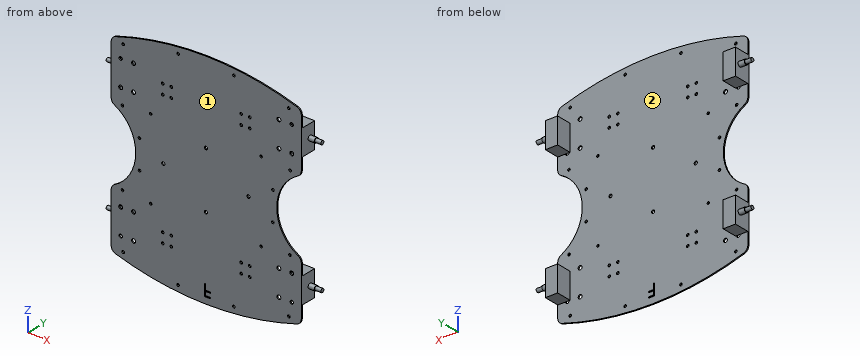
from build123d import *

# Parameters (mm, degrees)
SKETCH1_R           = 2.75
SKETCH1_R_2         = 3.19965974
SKETCH1_R_3         = 2.125
SKETCH1_R_4         = 2.6
SKETCH1_R_5         = 2
BOSS_EXTRUDE1_DEPTH = 2
CUT_EXTRUDE1_DEPTH  = 238.125138886
SKETCH3_R           = 2.125
CUT_EXTRUDE2_DEPTH  = 238.125138886
SKETCH5_W           = 42
SKETCH5_H           = 25
BOSS_EXTRUDE2_DEPTH = 20
BOSS_EXTRUDE3_START = -310
SKETCH5_2_W         = 42
SKETCH5_2_H         = 25
BOSS_EXTRUDE3_DEPTH = 20
SKETCH6_R           = 4
BOSS_EXTRUDE4_DEPTH = 10
SKETCH7_R           = 3
BOSS_EXTRUDE5_DEPTH = 10


with BuildPart() as part:
    # Sketch1 → Boss-Extrude1 (new body)
    with BuildSketch(Plane(origin=(0, 0, 0), x_dir=(1, 0, 0), z_dir=(0, 1, 0))):
        with BuildLine():
            Line((-155, 147.496205723), (-155, 66.522508221))
            ThreePointArc((-155, 66.522508221), (-153.570009292, 61.369359597), (-149.689011853, 57.690001904))
            ThreePointArc((-149.689011853, 57.690001904), (-115, 0), (-149.689011853, -57.690001904))
            ThreePointArc((-149.689011853, -57.690001904), (-153.570009292, -61.369359597), (-155, -66.522508221))
            Line((-155, -66.522508221), (-155, -147.496205723))
            ThreePointArc((-155, -147.496205723), (-153.049591193, -153.429508482), (-147.959183673, -157.048338049))
            ThreePointArc((-147.959183673, -157.048338049), (0, -179.441721715), (147.959183673, -157.048338049))
            ThreePointArc((147.959183673, -157.048338049), (153.049591193, -153.429508482), (155, -147.496205723))
            Line((155, -147.496205723), (155, -66.522508221))
            ThreePointArc((155, -66.522508221), (153.570009292, -61.369359597), (149.689011853, -57.690001904))
            ThreePointArc((149.689011853, -57.690001904), (115, 0), (149.689011853, 57.690001904))
            ThreePointArc((149.689011853, 57.690001904), (153.570009292, 61.369359597), (155, 66.522508221))
            Line((155, 66.522508221), (155, 147.496205723))
            ThreePointArc((155, 147.496205723), (153.049591193, 153.429508482), (147.959183673, 157.048338049))
            ThreePointArc((147.959183673, 157.048338049), (0, 179.441721715), (-147.959183673, 157.048338049))
            ThreePointArc((-147.959183673, 157.048338049), (-153.049591193, 153.429508482), (-155, 147.496205723))
        make_face()
        with Locations(Location((-139.47, 128.51, 0), (0, 0, 270))):
            Circle(SKETCH1_R, mode=Mode.SUBTRACT)
        with Locations(Location((-139.47, 86.51, 0), (0, 0, 270))):
            Circle(SKETCH1_R_2, mode=Mode.SUBTRACT)
        with Locations(Location((139.47, 86.51, 0), (0, 0, 270))):
            Circle(SKETCH1_R_2, mode=Mode.SUBTRACT)
        with Locations(Location((139.47, 128.51, 0), (0, 0, 270))):
            Circle(SKETCH1_R, mode=Mode.SUBTRACT)
        with Locations(Location((139.47, -86.51, 0), (0, 0, 270))):
            Circle(SKETCH1_R_2, mode=Mode.SUBTRACT)
        with Locations(Location((139.47, -128.51, 0), (0, 0, 270))):
            Circle(SKETCH1_R, mode=Mode.SUBTRACT)
        with Locations(Location((-139.47, -86.51, 0), (0, 0, 270))):
            Circle(SKETCH1_R_2, mode=Mode.SUBTRACT)
        with Locations(Location((-139.47, -128.51, 0), (0, 0, 270))):
            Circle(SKETCH1_R, mode=Mode.SUBTRACT)
        with Locations(Location((-70.97, 115.51, 0), (0, 0, 270))):
            Circle(SKETCH1_R_3, mode=Mode.SUBTRACT)
        with Locations(Location((-56.97, 115.51, 0), (0, 0, 270))):
            Circle(SKETCH1_R_3, mode=Mode.SUBTRACT)
        with Locations(Location((-70.97, 99.51, 0), (0, 0, 270))):
            Circle(SKETCH1_R_3, mode=Mode.SUBTRACT)
        with Locations(Location((-56.97, 99.51, 0), (0, 0, 270))):
            Circle(SKETCH1_R_3, mode=Mode.SUBTRACT)
        with Locations(Location((56.97, 99.51, 0), (0, 0, 270))):
            Circle(SKETCH1_R_3, mode=Mode.SUBTRACT)
        with Locations(Location((70.97, 99.51, 0), (0, 0, 270))):
            Circle(SKETCH1_R_3, mode=Mode.SUBTRACT)
        with Locations(Location((56.97, 115.51, 0), (0, 0, 270))):
            Circle(SKETCH1_R_3, mode=Mode.SUBTRACT)
        with Locations(Location((70.97, 115.51, 0), (0, 0, 270))):
            Circle(SKETCH1_R_3, mode=Mode.SUBTRACT)
        with Locations(Location((70.97, -99.51, 0), (0, 0, 270))):
            Circle(SKETCH1_R_3, mode=Mode.SUBTRACT)
        with Locations(Location((56.97, -99.51, 0), (0, 0, 270))):
            Circle(SKETCH1_R_3, mode=Mode.SUBTRACT)
        with Locations(Location((70.97, -115.51, 0), (0, 0, 270))):
            Circle(SKETCH1_R_3, mode=Mode.SUBTRACT)
        with Locations(Location((56.97, -115.51, 0), (0, 0, 270))):
            Circle(SKETCH1_R_3, mode=Mode.SUBTRACT)
        with Locations(Location((-56.97, -99.51, 0), (0, 0, 270))):
            Circle(SKETCH1_R_3, mode=Mode.SUBTRACT)
        with Locations(Location((-70.97, -99.51, 0), (0, 0, 270))):
            Circle(SKETCH1_R_3, mode=Mode.SUBTRACT)
        with Locations(Location((-56.97, -115.51, 0), (0, 0, 270))):
            Circle(SKETCH1_R_3, mode=Mode.SUBTRACT)
        with Locations(Location((-70.97, -115.51, 0), (0, 0, 270))):
            Circle(SKETCH1_R_3, mode=Mode.SUBTRACT)
        with Locations(Location((-118.47, 128.51, 0), (0, 0, 270))):
            Circle(SKETCH1_R_2, mode=Mode.SUBTRACT)
        with Locations(Location((-118.47, 86.51, 0), (0, 0, 270))):
            Circle(SKETCH1_R_2, mode=Mode.SUBTRACT)
        with Locations(Location((118.47, 86.51, 0), (0, 0, 270))):
            Circle(SKETCH1_R_2, mode=Mode.SUBTRACT)
        with Locations(Location((118.47, 128.51, 0), (0, 0, 270))):
            Circle(SKETCH1_R_2, mode=Mode.SUBTRACT)
        with Locations(Location((118.47, -128.51, 0), (0, 0, 270))):
            Circle(SKETCH1_R_2, mode=Mode.SUBTRACT)
        with Locations(Location((118.47, -86.51, 0), (0, 0, 270))):
            Circle(SKETCH1_R_2, mode=Mode.SUBTRACT)
        with Locations(Location((-118.47, -86.51, 0), (0, 0, 270))):
            Circle(SKETCH1_R_2, mode=Mode.SUBTRACT)
        with Locations(Location((-118.47, -128.51, 0), (0, 0, 270))):
            Circle(SKETCH1_R_2, mode=Mode.SUBTRACT)
        with Locations(Location((-0.51, 46.4, 0), (0, 0, 270))):
            Circle(SKETCH1_R_4, mode=Mode.SUBTRACT)
        with Locations(Location((68.99, -0.1, 0), (0, 0, 270))):
            Circle(SKETCH1_R_4, mode=Mode.SUBTRACT)
        with Locations(Location((-0.51, -46.6, 0), (0, 0, 270))):
            Circle(SKETCH1_R_4, mode=Mode.SUBTRACT)
        with Locations(Location((-70.01, -0.1, 0), (0, 0, 270))):
            Circle(SKETCH1_R_4, mode=Mode.SUBTRACT)
        with Locations(Location((-90.51, 64.9, 0), (0, 0, 270))):
            Circle(SKETCH1_R_5, mode=Mode.SUBTRACT)
        with Locations(Location((89.49, 64.9, 0), (0, 0, 270))):
            Circle(SKETCH1_R_5, mode=Mode.SUBTRACT)
        with Locations(Location((89.49, -65.1, 0), (0, 0, 270))):
            Circle(SKETCH1_R_5, mode=Mode.SUBTRACT)
        with Locations(Location((-90.51, -65.1, 0), (0, 0, 270))):
            Circle(SKETCH1_R_5, mode=Mode.SUBTRACT)
    extrude(amount=BOSS_EXTRUDE1_DEPTH)

    # Sketch2 → Cut-Extrude1 (cut, through all)
    with BuildSketch(Plane(origin=(0, 2, 0), x_dir=(1, 0, 0), z_dir=(0, 1, 0))):
        Polygon((-2.557692308, 169.05), (6.723076923, 169.05), (6.723076923, 167.096153846), (-0.848076923, 167.096153846), (-0.848076923, 161.234615385), (6.723076923, 161.234615385), (6.723076923, 159.280769231), (-0.848076923, 159.280769231), (-0.848076923, 150), (-2.557692308, 150), align=None)
    extrude(amount=-CUT_EXTRUDE1_DEPTH, mode=Mode.SUBTRACT)

    # Sketch3 → Cut-Extrude2 (cut, through all)
    with BuildSketch(Plane(origin=(0, 2, 0), x_dir=(1, 0, 0), z_dir=(0, 1, 0))):
        with Locations(Location((-135.418169234, 150.357764594, 0), (0, 0, 270))):
            Circle(SKETCH3_R)
        with Locations(Location((-45.914062128, 167.285855531, 0), (0, 0, 270))):
            Circle(SKETCH3_R)
        with Locations(Location((45.176775579, 167.354684187, 0), (0, 0, 270))):
            Circle(SKETCH3_R)
        with Locations(Location((134.706362354, 150.561871932, 0), (0, 0, 270))):
            Circle(SKETCH3_R)
        with Locations(Location((134.706362354, -150.561871932, 0), (0, 0, 90))):
            Circle(SKETCH3_R)
        with Locations(Location((45.176775579, -167.354684187, 0), (0, 0, 90))):
            Circle(SKETCH3_R)
        with Locations(Location((-45.914062128, -167.285855531, 0), (0, 0, 90))):
            Circle(SKETCH3_R)
        with Locations(Location((-135.418169234, -150.357764594, 0), (0, 0, 90))):
            Circle(SKETCH3_R)
        with Locations(Location((-136.498269922, 61.257473969, 0), (0, 0, 270))):
            Circle(SKETCH3_R)
        with Locations(Location((-108.723114922, 23.387075934, 0), (0, 0, 270))):
            Circle(SKETCH3_R)
        with Locations(Location((-108.785429276, -23.5769784, 0), (0, 0, 270))):
            Circle(SKETCH3_R)
        with Locations(Location((-136.660983133, -61.373536175, 0), (0, 0, 270))):
            Circle(SKETCH3_R)
        with Locations(Location((136.660983133, -61.373536175, 0), (0, 0, 90))):
            Circle(SKETCH3_R)
        with Locations(Location((108.785429276, -23.5769784, 0), (0, 0, 90))):
            Circle(SKETCH3_R)
        with Locations(Location((108.723114922, 23.387075934, 0), (0, 0, 90))):
            Circle(SKETCH3_R)
        with Locations(Location((136.498269922, 61.257473969, 0), (0, 0, 90))):
            Circle(SKETCH3_R)
    extrude(amount=-CUT_EXTRUDE2_DEPTH, mode=Mode.SUBTRACT)

    # Sketch5 → Boss-Extrude2 (add)
    with BuildSketch(Plane.ZY.offset(155)):
        with Locations((-107.009356972, 14.5)):
            Rectangle(SKETCH5_W, SKETCH5_H)
        with Locations((107.009356972, 14.5)):
            Rectangle(SKETCH5_W, SKETCH5_H)
    extrude(amount=-BOSS_EXTRUDE2_DEPTH)

    # Sketch5<2> → Boss-Extrude3 (add)
    with BuildSketch(Plane.ZY.offset(155).offset(BOSS_EXTRUDE3_START)):
        with Locations((-107.009356972, 14.5)):
            Rectangle(SKETCH5_2_W, SKETCH5_2_H)
        with Locations((107.009356972, 14.5)):
            Rectangle(SKETCH5_2_W, SKETCH5_2_H)
    extrude(amount=BOSS_EXTRUDE3_DEPTH)

    # Sketch6 → Boss-Extrude4 (add)
    with BuildSketch(Plane.ZY.offset(155)):
        with Locations(Location((107.009356972, 17.75, 0), (0, 0, 180))):
            Circle(SKETCH6_R)
        with Locations(Location((-107.009356972, 17.75, 0), (0, 0, 180))):
            Circle(SKETCH6_R)
    boss_extrude4 = extrude(amount=BOSS_EXTRUDE4_DEPTH)

    # Sketch7 → Boss-Extrude5 (add)
    with BuildSketch(Plane.ZY.offset(165)):
        with Locations((107.009356972, 17.75)):
            Circle(SKETCH7_R)
        with Locations((-107.009356972, 17.75)):
            Circle(SKETCH7_R)
    boss_extrude5 = extrude(amount=BOSS_EXTRUDE5_DEPTH)

    # Mirror1: Boss-Extrude4, Boss-Extrude5 across plane
    add(boss_extrude4.mirror(Plane.ZY))
    add(boss_extrude5.mirror(Plane.ZY))


solid = part.part
Geometry: final body of the model. Coordinates: model frame, mm. Face numbers are marked on the shaded views. Coordinates: 2 decimals unless noted, no trailing zeros. Order: outer loops, then holes, each group sorted by start corner. A loop starts at its lowest first (then second) coordinate and runs counter-clockwise, first axis right, second up. Notation, with made-up numbers: M 76,4.5 L 122,4.5 A18 ccw 122,11.5 Z; hole C 86,88.25 d4. An arc over 180 degrees is marked long. One line per question, with ' | ' between items. Start each with the question number.
Item 1: Pin query (flat end, axial travel): pin 1 Ø2.5 at (x, z) = (-70.97, -115.51) entering from -Y; pin 2 Ø5 at (x, z) = (-56.97, -115.51) entering from +Y; pin 3 Ø8 at (y, z) = (12.5, 120) entering from -X; pin 4 Ø4 at (x, y) = (136.5, 9) entering from -Z. Return the tip coordinate at first contact, or that it passes through.
Item 2: Ray query, probe 1 along X at (y, z) = (0.8, 0.1); probe 2 along X at (y, z) = (0.6, 115.51) (3 decimals); probe 3 along X at (y, z) = (1.2, 86.51). Return the intervals inside material, ascending. Write a range as [from, to].
Item 3: Cut plane A-A, the plane y = 7.75. Return the cut outline in (x, z), then the cut area to 3 significant figures.
Item 4: Draft query along X for the marked faces 1 and 2. Return one class per face: released by +X, released by -X, zero draft, split by the parting line, or undercut.
Item 5: Cut plane B-B, the plane x = -20. Return the cut outline in (y, z), then the cut area to 3 significant figures.
A:
1) pin 1: passes through | pin 2: stops at y = 2 | pin 3: stops at x = -155 | pin 4: stops at z = -128.01
2) probe 1: x = [-115, -72.61], [-67.41, 66.39], [71.59, 115] | probe 2: x = [-155, -73.095], [-68.845, -59.095], [-54.845, 54.845], [59.095, 68.845], [73.095, 155] | probe 3: x = [-155, -142.67], [-136.27, -121.67], [-115.27, 115.27], [121.67, 136.27], [142.67, 155]
3) outline: M -155,-128.01 L -135,-128.01 L -135,-86.01 L -155,-86.01 Z; M -155,86.01 L -135,86.01 L -135,128.01 L -155,128.01 Z; M 135,-128.01 L 155,-128.01 L 155,-86.01 L 135,-86.01 Z; M 135,86.01 L 155,86.01 L 155,128.01 L 135,128.01 Z | area: 3,360 mm2
4) face 1: zero draft | face 2: undercut
5) outline: M 0,-179.04 L 2,-179.04 L 2,179.04 L 0,179.04 Z | area: 716 mm2
